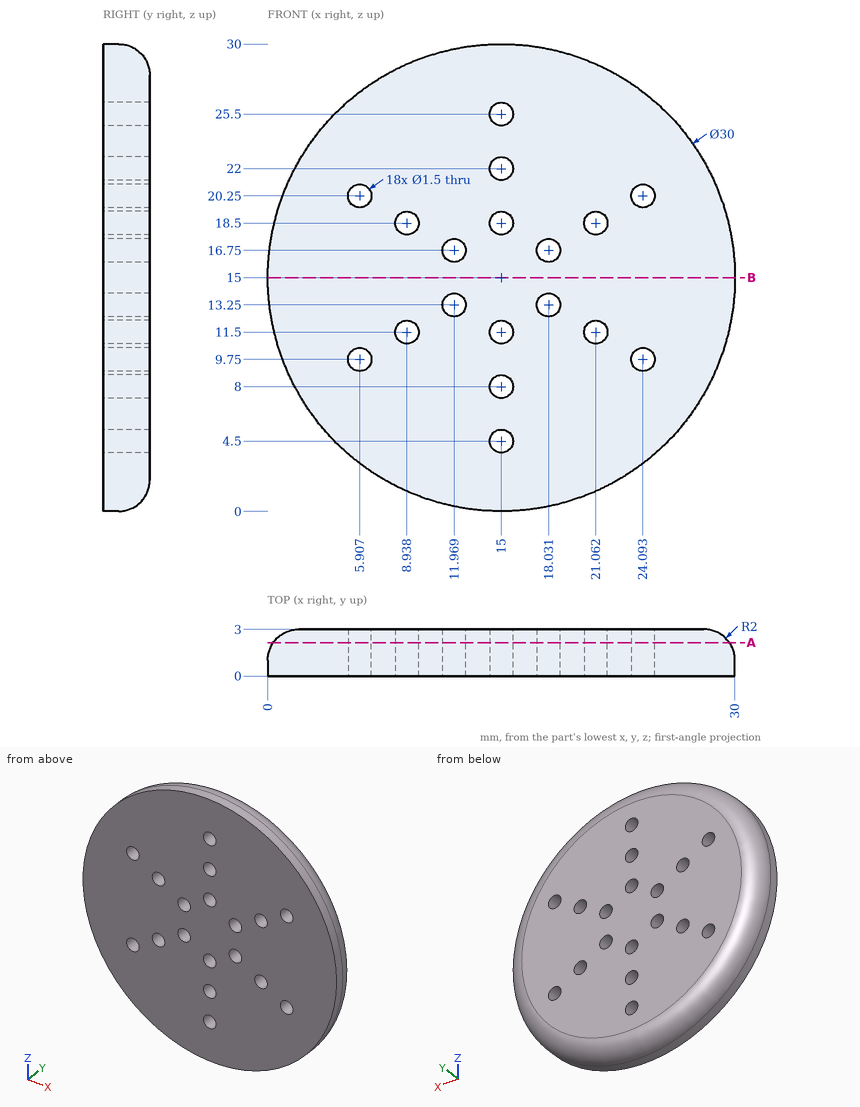
Input: dimensioned drawing with shaded views. Units: mm. Origin: part minimum x, y, z. Give positions to 0.01 mm unless a question says otherwise; leave off trailing zeros. Write each loop counter-clockwise with the first axis right and the second up, starting at its lowest first coordinate (ties: lowest second). Pieces come first, ordered by that corner, then holes. Notation, with made-up numbers: (-5, -19) -> (0, -19) arc R24 cw to (0, -1) -> close; hole circle Ø6 at (44, 14.25). An arc over 180 degrees is marked (long way). Answer as a JSON object with one key per item and string values.
1. Cut plane B-B on z = 15. Output: boundary loops of the cut face in (x, y).
Ans:
{"outline": "(0, 0) -> (30, 0) -> (30, 1) arc R2 ccw to (28, 3) -> (2, 3) arc R2 ccw to (0, 1) -> close"}
2. Ray query, probe 1 along X at (y, z) = (0.2, 18); probe 2 along X at (y, z) = (1.3, 9.75); probe 3 along Z at (x, y) = (17.5, 2.35). Return the intervals inside material, ascending. Write a range as from..to.
Ans:
{"probe 1": "x = 0.3..8.38, 9.5..14.44, 15.56..20.5, 21.62..29.7", "probe 2": "x = 0.97..5.16, 6.66..23.34, 24.84..29.03", "probe 3": "z = 0.74..12.72, 13.78..16.22, 17.28..29.26"}
3. Contact query for a flat-ended pin moving along its axis: pin 1 (1 mm diameter, centred on y = 0.5, z = 8, fed in from -X). Output: stop coordinate, or through.
Ans:
{"pin 1": "stops at x = 1.48"}
4. Cut plane A-A on y = 2.15. Count the separate pieces of the cut face and the enclosed holes in it, and give its area (3 significant figures).
Ans:
{"separate pieces": "1", "enclosed holes": "18", "area": "641 mm^2"}
